```python
from build123d import *

# Parameters (mm, degrees)
BOSS_EXTRUDE1_DEPTH   = 19.05
F_6_CLEARANCE_HOLE1_D = 3.7973


with BuildPart() as part:
    # Sketch1 → Boss-Extrude1 (new body)
    with BuildSketch(Plane.XY):
        with BuildLine():
            Line((6.074664, 12.7), (-3.876684639, 5.029295797))
            ThreePointArc((-3.876684639, 5.029295797), (-5.029295797, -3.876684639), (3.876684639, -5.029295797))
            Line((3.876684639, -5.029295797), (26.877233079, 12.7))
            Line((26.877233079, 12.7), (6.074664, 12.7))
        make_face()
    extrude(amount=BOSS_EXTRUDE1_DEPTH)

    # #6 Clearance Hole1 (through all)
    with Locations(Plane.XY.offset(19.05)):
        with Locations((0, 0)):
            Hole(F_6_CLEARANCE_HOLE1_D / 2)


solid = part.part
```
Work out the finished part from the listing and answer in its coordinate system (mm). Give positions to 0.01 mm unless a question says otherwise; leave off trailing zeros. Order: outer loops, then holes, each group sorted by start corner. A loop starts at its lowest first (then second) coordinate and runs counter-clockwise, first axis right, second up.
1. The mould has two halves that part along X. Classify faces 1 (the flat face through (6, 5, 0)), 2 (the cylindrical face through (-1.8, 0.6, 9.4)), 3 (the cylindrical face through (-5.11, -3.77, 9.39)): released by +X, released by -X, zero draft, split by the parting line, or undercut.
Result sheet:
face 1: zero draft
face 2: undercut
face 3: split by the parting line
2. Straight lines are drawn through the part: L1, parallel to X at y = -0.5, z = 8.25; L2, parallel to Y at x = 0, z = 12; L3, parallel to X at y = -1, z = 3. For each, find the intervals that lie inside material, in ascending order.
Result sheet:
L1: x = -6.33 to -1.83, 1.83 to 9.75
L2: y = -6.35 to -1.9, 1.9 to 8.02
L3: x = -6.27 to -1.61, 1.61 to 9.1
3. Section B-B, the plane x = 0 is taken. Determine the outline of the cut face in (y, z).
Result sheet:
outline: (-6.35, 0) - (-1.9, 0) - (-1.9, 19.05) - (-6.35, 19.05) - close; (1.9, 0) - (8.02, 0) - (8.02, 19.05) - (1.9, 19.05) - close
4. Section D-D, the plane y = 4.25 is taken. Determine the outline of the cut face in (x, z), and give its area (3 significant figures).
Result sheet:
outline: (-4.72, 0) - (15.91, 0) - (15.91, 19.05) - (-4.72, 19.05) - close
area: 393 mm2
5. Section A-A, the plane y = 0.5 is taken. Determine the outline of the cut face in (x, z), and give its area (3 significant figures).
Result sheet:
outline: (-6.33, 0) - (-1.83, 0) - (-1.83, 19.05) - (-6.33, 19.05) - close; (1.83, 0) - (11.05, 0) - (11.05, 19.05) - (1.83, 19.05) - close
area: 261 mm2
6. Section C-C, the plane z = 11.75 is taken. Determine the outline of the cut face in (x, y).
Result sheet:
outline: (-3.88, 5.03) arc R6.35 ccw to (3.88, -5.03) - (26.88, 12.7) - (6.07, 12.7) - close; hole circle Ø3.8 at (0, 0)
7. Each of these flat-tipped pins is pushed along its axis until it touches: P1, Ø1, axis at y = 2.5, z = 7, coming from the -X side; P2, Ø3, axis at x = -2.5, z = 2.5, coming from the -Y side; P3, Ø1, axis at y = 1, z = 4.5, coming from the -X side. Where does it stop, or does it pass through?
Result sheet:
P1: stops at x = -6.03
P2: stops at y = -6.27
P3: stops at x = -6.33
